Autodesk Fusion 360 part; units mm, degrees
sketch "Sketch1" plane through (0, 0, 0) normal (1, 0, 0) x (0, 1, 0)
  line L0 (9.5131, 10.735) -> (-5.4869, 10.735)
  line L1 (-5.4869, 10.735) -> (-5.4869, -4.265)
  line L2 (-5.4869, -4.265) -> (9.5131, -4.265)
  line L3 (9.5131, -4.265) -> (9.5131, 10.735)
  line L4 (9.5131, 10.735) -> (-5.4869, -4.265) construction
  line L5 (-5.4869, 10.735) -> (9.5131, -4.265) construction
  line L6 (8.0131, -2.765) -> (-3.9869, -2.765)
  line L7 (-3.9869, -2.765) -> (-3.9869, 9.235)
  line L8 (-3.9869, 9.235) -> (8.0131, 9.235)
  line L9 (8.0131, 9.235) -> (8.0131, -2.765)
  line L10 (8.0131, -2.765) -> (-3.9869, 9.235) construction
  line L11 (-3.9869, -2.765) -> (8.0131, 9.235) construction
  point P0 (2.0131, 3.235)
  point P1 (2.0131, 3.235)
  dimension "d3" = 15
  dimension "d4" = 15
  dimension "d5" = 12
  dimension "d6" = 12
extrude "Extrude1" add sketch "Sketch1" along normal blind 5
sketch "Sketch2" plane through (5, 0, 0) normal (1, 0, 0) x (0, 1, 0)
  line L0 (-3.9869, 9.235) -> (8.0131, 9.235)
  line L1 (8.0131, 9.235) -> (8.0131, -2.765)
  line L2 (8.0131, -2.765) -> (-3.9869, -2.765)
  line L3 (-3.9869, -2.765) -> (-3.9869, 9.235)
  line L4 (9.5131, -4.265) -> (9.5131, 10.735)
  line L5 (9.5131, 10.735) -> (-5.4869, 10.735)
  line L6 (-5.4869, 10.735) -> (-5.4869, -4.265)
  line L7 (-5.4869, -4.265) -> (9.5131, -4.265)
  line L8 (17.0131, 18.235) -> (-12.9869, -11.765) construction
  line L9 (-12.9869, 18.235) -> (17.0131, -11.765) construction
  circle A0 centre (14.5131, 15.735) radius 1.6
  circle A1 centre (-10.4869, 15.735) radius 1.6
  circle A2 centre (-10.4869, -9.265) radius 1.6
  circle A3 centre (14.5131, -9.265) radius 1.6
  circle A4 centre (-10.4869, 15.735) radius 3.1
  circle A5 centre (14.5131, 15.735) radius 3.1
  circle A6 centre (-10.4869, -9.265) radius 3.1
  line L10 (9.5131, 10.735) -> (-5.4869, 10.735)
  line L11 (-5.4869, 10.735) -> (-5.4869, -4.265)
  line L12 (-5.4869, -4.265) -> (9.5131, -4.265)
  line L13 (9.5131, -4.265) -> (9.5131, 10.735)
  line L14 (9.5131, 10.735) -> (-5.4869, -4.265) construction
  line L15 (-5.4869, 10.735) -> (9.5131, -4.265) construction
  line L16 (-8.7038, 18.2708) -> (2.0131, 10.735)
  line L17 (2.0131, 10.735) -> (12.73, 18.2708)
  line L18 (-13.0227, 13.9519) -> (-5.4869, 3.235)
  line L19 (-5.4869, 3.235) -> (-13.0227, -7.4819)
  line L20 (-8.7038, -11.8008) -> (2.0131, -4.265)
  line L21 (9.5131, 3.235) -> (17.0489, 13.9519)
  circle A7 centre (14.5131, -9.265) radius 3.1
  line L22 (9.5131, 3.235) -> (17.0489, -7.4819)
  line L23 (2.0131, -4.265) -> (12.73, -11.8008)
  point P0 (2.0131, 3.235)
  point P1 (2.0131, 3.235)
  point P2 (2.0131, 3.235)
  dimension "d11" = 3.2
  dimension "d12" = 12.5
  dimension "d13" = 3.2
  dimension "d14" = 3.2
  dimension "d15" = 3.2
  dimension "d17" = 25
  dimension "d18" = 12.5
  dimension "d19" = 25
  dimension "d20" = 6.2
  dimension "d21" = 6.2
  dimension "d22" = 6.2
  dimension "d23" = 6.2
extrude "Extrude2" add sketch "Sketch2" along normal blind 3
extrude "Extrude4" add sketch "Sketch1" against normal blind 5
extrude "Extrude3" [suppressed]
equation "d11 = motorScrewHole"
equation "d13 = motorScrewHole"
equation "d14 = motorScrewHole"
equation "d15 = motorScrewHole"
equation "motorScrewHole = 3.2 mm"
equation "d20 = motorScrewHole + 3 mm"
equation "d21 = motorScrewHole + 3 mm"
equation "d22 = motorScrewHole + 3 mm"
equation "d23 = motorScrewHole + 3 mm"
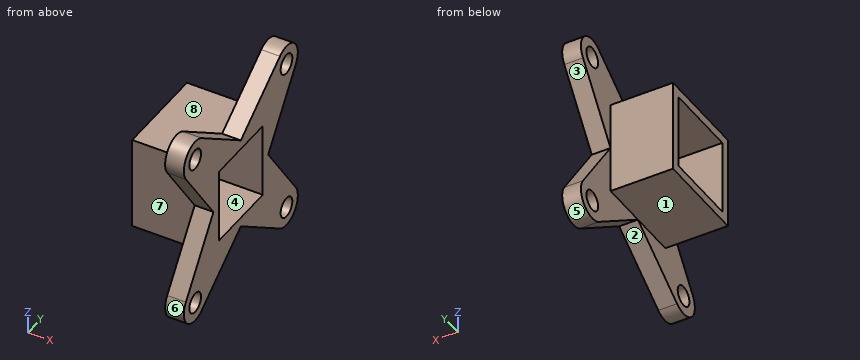
Design review of the part built by this model. Coordinates are the model's own, in mm. Face numbers are marked on the shaded views. A direction names the side the tool comes from. Coordinates: 2 decimals unless noted, no trailing zeros. Order: outer loops, then holes, each group sorted by start corner. A loop starts at its lowest first (then second) coordinate and runs counter-clockwise, first axis right, second up.
1) Take a section at B-B, the plane z = 4.5. Give the boundary of the cut face in (x, y), and give its area (3 significant figures).
2) Clearance check with flat-ended pins moving along their axes: pin 1 (5 mm diameter, centred on x = 0.5, y = 0.5, fed in from +Z) (3 decimals); pin 2 (6 mm diameter, centred on x = 4.5, z = 5.5, fed in from +Y); pin 3 (2 mm diameter, centred on x = 5, z = -4, fed in from -Y). State where each tip first meets the part, or that it passes through.
3) Mouldability with a two-part tool opening along Z and no side actions: class the marked faces 5, 6, 7 and 8 as +Z half, -Z half, draft (parallel to the pull), parting line (faces both ways), or undercut.
4) Take a section at D-D, the plane y = -3.5. Give the boundary of the cut face in (x, z) (3 decimals), and give its area (3 significant figures).
5) Take a section at C-C, the plane y = 15. Give the boundary of the cut face in (x, z), and give its area (3 significant figures).
6) For the marked faces 1, 2, 3 and 4, list the 3-axis set-ups (+Z, -Z, +X, -X, +Y, -Y) from which the entire face can be reached by the end or side of a thin tool; tool diameter is ignored.
7) Take a section at A-A, the plane x = 1.5. Give the boundary of the cut face in (y, z) (3 decimals).
8) Wall thickness on line 1 along Z through (x, y) = (-0.75, 5) (3 decimals); line 2 along Y through (x, z) = (1, 9); line 3 along X through (y, z) = (-9, 15): over which ranges is each line inside the solid? List them lowest first.
Returned:
1. outline: (-5, -5.49) - (5, -5.49) - (5, -6.38) - (8, -6.38) - (8, -3.99) - (-5, -3.99) - close; (-5, 8.01) - (8, 8.01) - (8, 10.4) - (5, 10.4) - (5, 9.51) - (-5, 9.51) - close
1. area: 44.3 mm2
2. pin 1: stops at z = 10.735
2. pin 2: stops at y = 13.19
2. pin 3: stops at y = -11.28
3. face 5: undercut
3. face 6: undercut
3. face 7: draft
3. face 8: +Z half
4. outline: (-5, -4.265) - (5, -4.265) - (5, -8.142) - (8, -8.142) - (8, -2.765) - (-5, -2.765) - close; (-5, 9.235) - (8, 9.235) - (8, 14.612) - (5, 14.612) - (5, 10.735) - (-5, 10.735) - close
4. area: 62.3 mm2
5. outline: (5, -12.33) - (8, -12.33) - (8, -10.79) - (5, -10.79) - close; (5, -7.74) - (8, -7.74) - (8, -4.57) - (5, -4.57) - close; (5, 11.04) - (8, 11.04) - (8, 14.21) - (5, 14.21) - close; (5, 17.26) - (8, 17.26) - (8, 18.8) - (5, 18.8) - close
5. area: 28.3 mm2
6. face 1: -Z, -X, +Y, -Y
6. face 2: -Z, +X, -X
6. face 3: +X, -X, +Y
6. face 4: +X, -X
7. outline: (-5.487, -4.265) - (9.513, -4.265) - (9.513, 10.735) - (-5.487, 10.735) - close; hole (-3.987, -2.765) - (8.013, -2.765) - (8.013, 9.235) - (-3.987, 9.235) - close
8. line 1: z = -4.265 to -2.765, 9.235 to 10.735
8. line 2: y = -5.49 to -3.99, 8.01 to 9.51
8. line 3: x = 5 to 8
